Work out the finished part from the listing and answer in its coordinate system (mm). Face numbers are marked on the shaded views. Coordinates: 2 decimals unless noted, no trailing zeros. Write each loop counter-clockwise with the first axis right and the second up, starting at its lowest first coordinate (ties: lowest second). Pieces come first, ordered by that corner, then holes. Notation, with made-up numbers: (75, -25.5) - (86, -25.5) arc R21 cw to (86, -6.5) - close; hole circle Ø8 at (34.25, 1.5). An arc over 180 degrees is marked (long way). Use one line per item in the form item = value. Start each with the question number.
Item 1: A cutting plane is placed at B-B (z = -35). Write down the section's boundary in (x, y), then the cut area to 3 significant figures.
Item 2: Determine the mould class of the marked faces 1, 2 and 3 for opening direction X: released by +X, released by -X, zero draft, split by the parting line, or undercut.
Item 3: A cutting plane is placed at D-D (x = 11). Write down the section's boundary in (y, z).
Item 4: A cutting plane is placed at C-C (x = -28). Write down the section's boundary in (y, z), then the cut area to 3 significant figures.
Item 5: Consider probe 1 along Z at (x, y) = (-38, -31); probe 2 along X at (y, z) = (88.5, -29.5); probe 3 along X at (y, z) = (-82.5, 0.5). Determine where each line is inside the solid, lowest interval first.
Item 6: Given pin 1 (15 mm diameter, centred on x = 11.5, z = -30.5, fed in from -Y); pin 2 (2.5 mm diameter, centred on y = 4.5, z = 1.5, fed in from +X); pin 3 (2 mm diameter, centred on x = -34, z = -6.5, fed in from -Y), each flat-ended and moving along its own axis, determine where each tip first touches the part or whether it passes through.
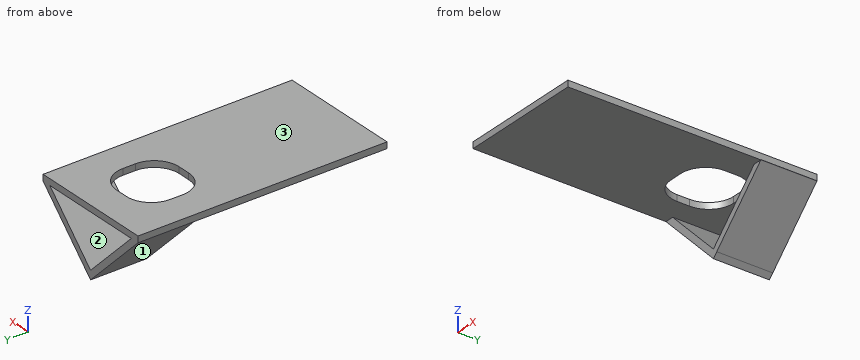
Autodesk Inventor part; units mm, degrees
ref_plane "YZ Plane" through (0, 0, 0) normal (1, 0, 0) x (0, 1, 0)
ref_plane "XZ Plane" through (0, 0, 0) normal (0, 1, 0) x (-1, 0, 0)
ref_plane "XY Plane" through (0, 0, 0) normal (0, 0, 1) x (1, 0, 0)
sketch "Sketch1" plane through (0, 0, 0) normal (0, 0, 1) x (1, 0, 0)
  line L0 (-50, -100) -> (50, -100)
  line L1 (50, -100) -> (50, 100)
  line L2 (50, 100) -> (-50, 100)
  line L3 (-50, 100) -> (-50, -100)
  line L4 (-50, -100) -> (50, 100) construction
  line L5 (50, -100) -> (-50, 100) construction
  point P0 (0, 0)
  dimension "d0" = 100
  dimension "d1" = 200
extrude "Extrusion1" add sketch "Sketch1" along normal blind 5
sketch "Sketch2" plane through (-50, 100, 0) normal (0, 1, 0) x (1, 0, 0)
  line L0 (0, 0) -> (100, 0)
  line L1 (0, 0) -> (49.9986, 49.9986)
  line L2 (49.9986, 49.9986) -> (53.5341, 46.463)
  line L3 (53.5341, 46.463) -> (3.5355, -3.5355)
  line L4 (3.5355, -3.5355) -> (0, 0)
  line L5 (0, 0) -> (70.7086, 0) construction
  line L6 (100.108, -0.1109) -> (53.5341, 46.463)
  line L7 (53.5341, 46.463) -> (49.9986, 42.9275)
  line L8 (49.9986, 42.9275) -> (96.5724, -3.6464)
  line L9 (96.5724, -3.6464) -> (100.108, -0.1109)
  point P0 (50, 0)
  point P1 (49.9986, 42.9275)
  dimension "d4" = 45
  dimension "d5" = 5
  dimension "d6" = 5
extrude "Extrusion2" add sketch "Sketch2" against normal blind 45 contours L1 L2 L3 L0 | L0 L3 L4 | L8 L3 L6 L0 | L0 L6 L9 L8
sketch "Sketch6" plane through (0, 0, 5) normal (0, 0, 1) x (1, 0, 0)
  line L0 (4.9986, 75) -> (-5.0014, 75)
  line L1 (-25.0014, 55) -> (-25.0014, 45)
  line L2 (-5.0014, 25) -> (4.9986, 25)
  line L3 (24.9986, 45) -> (24.9986, 55)
  line L4 (24.9986, 75) -> (-25.0014, 25) construction
  line L5 (-25.0014, 75) -> (24.9986, 25) construction
  arc A0 (4.9986, 25) -> (24.9986, 45) centre (4.9986, 45) ccw
  arc A1 (24.9986, 55) -> (4.9986, 75) centre (4.9986, 55) ccw
  arc A2 (-5.0014, 75) -> (-25.0014, 55) centre (-5.0014, 55) ccw
  arc A3 (-25.0014, 45) -> (-5.0014, 25) centre (-5.0014, 45) ccw
  point P0 (0, 0)
  point P1 (-0.0014, 50)
  dimension "d21" = 50
  dimension "d22" = 50
  dimension "d23" = 20
extrude "Extrusion6" cut sketch "Sketch6" against normal blind 5
properties part number "fixation_v04b"
Answer:
q1.outline = (-15, 55) - (-7.93, 55) - (-7.93, 100) - (-15, 100) - close; (7.93, 55) - (15, 55) - (15, 100) - (7.93, 100) - close
q1.area = 636 mm²
q2.face_1 = released by -X
q2.face_2 = undercut
q2.face_3 = zero draft
q3.outline = (-100, 0) - (25.92, 0) - (25.92, 5) - (-100, 5) - close; (55, -39) - (100, -39) - (100, -31.93) - (55, -31.93) - close; (74.08, 0) - (100, 0) - (100, 5) - (74.08, 5) - close
q4.outline = (-100, 0) - (100, 0) - (100, 5) - (-100, 5) - close; (55, -22) - (100, -22) - (100, -14.93) - (55, -14.93) - close
q4.area = 1,320 mm²
q5.probe_1 = 0 to 5
q5.probe_2 = -20.5 to -13.43, 13.43 to 20.5
q5.probe_3 = -50 to 50
q6.pin_1 = 55
q6.pin_2 = 50
q6.pin_3 = through
